Input: dimensioned drawing with shaded views. Units: mm. Origin: part minimum x, y, z. A direction names the side the tool comes from. Give positions to 0.01 mm unless a question says otherwise; leave off trailing zeros. Order: outer loops, then holes, each group sorted by start corner. A loop starts at its lowest first (then second) coordinate and runs counter-clockwise, first axis right, second up. Notation, with made-up numbers: (38.5, 54.5) - (49.5, 54.5) arc R21 ccw to (49.5, 79.5) - close; hole circle Ø4 at (0.25, 33). An arc over 180 degrees is marked (long way). Use a Markdown table: item, result.
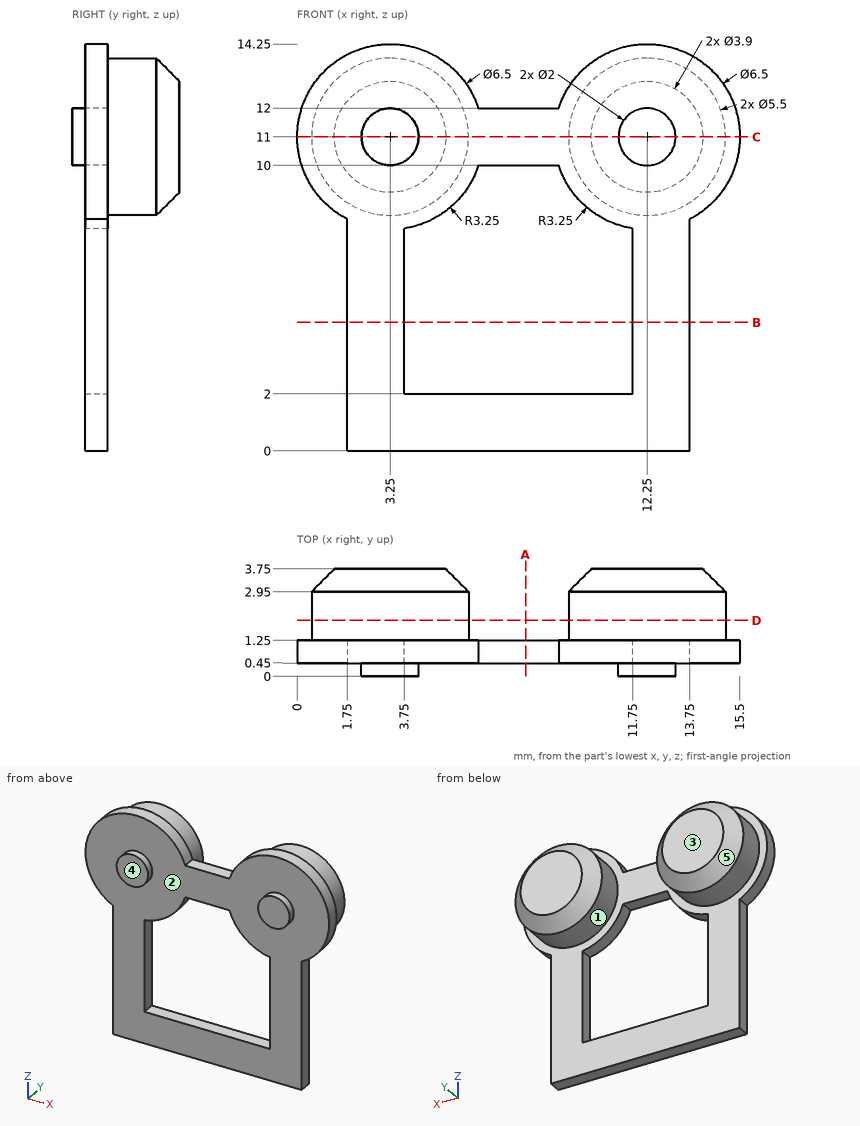
1. Section query D-D (y = 1.95). Return loops of the section in (x, z), then the cut area to 3 significant figures.
Response:
| item | result |
|---|---|
| outline | circle Ø5.5 at (3.25, 11); circle Ø5.5 at (12.25, 11) |
| area | 47.5 mm^2 |
2. Mould query, pull axis X, two halves, no side actions, for the marked faces 4 and 5. Classes: pulls with the +X half, pulls with the -X half, needs draft (parallel to the pull), parting line crosses it, or undercut.
Response:
| item | result |
|---|---|
| face 4 | needs draft |
| face 5 | undercut |
3. Set-up query: the marked faces 1, 2 and 3. Return all of +Z, -Z, +X, -X, +Y, -Y with unobstructed straight access to the full face (end or side cutting, diameter ignored); none if empty.
Response:
| item | result |
|---|---|
| face 1 | +Y |
| face 2 | -Y |
| face 3 | +Z, -Z, +X, -X, +Y |
4. Section query A-A (x = 8). Return loops of the section in (y, z), then the cut area to 3 significant figures.
Response:
| item | result |
|---|---|
| outline | (0.45, 0) - (1.25, 0) - (1.25, 2) - (0.45, 2) - close; (0.45, 10) - (1.25, 10) - (1.25, 12) - (0.45, 12) - close |
| area | 3.20 mm^2 |
5. Section query C-C (z = 11). Return loops of the section in (x, y).
Response:
| item | result |
|---|---|
| outline | (0, 0.45) - (2.25, 0.45) - (2.25, 0) - (4.25, 0) - (4.25, 0.45) - (11.25, 0.45) - (11.25, 0) - (13.25, 0) - (13.25, 0.45) - (15.5, 0.45) - (15.5, 1.25) - (15, 1.25) - (15, 2.95) - (14.2, 3.75) - (10.3, 3.75) - (9.5, 2.95) - (9.5, 1.25) - (6, 1.25) - (6, 2.95) - (5.2, 3.75) - (1.3, 3.75) - (0.5, 2.95) - (0.5, 1.25) - (0, 1.25) - close |
6. Material intervals for line 1 along X through (y, z) = (0.95, 1.25); line 2 along Y through (x, z) = (2, 8.5); line 3 along X through (y, z) = (1.4, 13.5), sorted ascending.
Response:
| item | result |
|---|---|
| line 1 | x = 1.75 to 13.75 |
| line 2 | y = 0.45 to 1.25 |
| line 3 | x = 2.1 to 4.4, 11.1 to 13.4 |
7. Section query B-B (z = 4.5). Return loops of the section in (x, y), then the cut area to 3 significant figures.
Response:
| item | result |
|---|---|
| outline | (1.75, 0.45) - (3.75, 0.45) - (3.75, 1.25) - (1.75, 1.25) - close; (11.75, 0.45) - (13.75, 0.45) - (13.75, 1.25) - (11.75, 1.25) - close |
| area | 3.20 mm^2 |
8. Pin query (flat end, axial travel): pin 1 (4 mm diameter, centred on x = 7.5, z = 5.5, fed in from +Y); pin 2 (0.9 mm diameter, centred on y = 1, z = 3, fed in from -X); pin 3 (7 mm diameter, centred on x = 10.5, z = 6.5, fed in from -Y); pin 4 (2 mm diameter, centred on x = 5.5, y = 3, fed in from -Z). Return the tip coordinate at first contact, or that it passes through.
Response:
| item | result |
|---|---|
| pin 1 | passes through |
| pin 2 | stops at x = 1.75 |
| pin 3 | stops at y = 0.45 |
| pin 4 | stops at z = 8.55 |
